from build123d import *

# Parameters (mm, degrees)
SKETCH1_W                    = 26.140328994
SKETCH1_H                    = 20
BASE_FLANGE1_DEPTH           = 3.175
EDGE_FLANGE1_STRIP_W         = 14.7
EDGE_FLANGE1_STRIP_H         = 3.175
EDGE_FLANGE1_STRIP_CUT_DEPTH = 20
EDGE_FLANGE1_DEPTH           = 20
EDGE_FLANGE2_STRIP_W         = 14.7
EDGE_FLANGE2_STRIP_H         = 3.175
EDGE_FLANGE2_STRIP_CUT_DEPTH = 20
EDGE_FLANGE2_DEPTH           = 20
FILLET1_R                    = 3
SKETCH18_R                   = 2.54
CUT_EXTRUDE2_DEPTH           = 360.816616057
SKETCH19_R                   = 2.54
CUT_EXTRUDE3_DEPTH           = 360.466065193


# Sheet-metal steps are written as plain solids
with BuildPart() as part:
    # Sketch1 → Base-Flange1 (new body)
    with BuildSketch(Plane.XY.offset(-1949.683434301)):
        with Locations((87.899449082, 311.128054742)):
            Rectangle(SKETCH1_W, SKETCH1_H)
    extrude(amount=BASE_FLANGE1_DEPTH)

    # Edge-Flange1 strip (across the edge) → Edge-Flange1 strip cut (cut)
    with BuildSketch(Plane(origin=(100.969613579, 321.128054742, -1949.683434301), x_dir=(-1, 0, 0), z_dir=(0, -1, 0))):
        with Locations((-6.35, -1.5875)):
            Rectangle(EDGE_FLANGE1_STRIP_W, EDGE_FLANGE1_STRIP_H)
    extrude(amount=EDGE_FLANGE1_STRIP_CUT_DEPTH, mode=Mode.SUBTRACT)

    # Edge-Flange1 section (across the edge) → Edge-Flange1 (add)
    with BuildSketch(Plane(origin=(100.969613579, 321.128054742, -1949.683434301), x_dir=(-1, 0, 0), z_dir=(0, -1, 0))):
        with BuildLine():
            Line((-3.175, 1), (-3.175, 34.9454))
            Line((-3.175, 34.9454), (0, 34.9454))
            Line((0, 34.9454), (0, 1))
            ThreePointArc((0, 1), (0.292893219, 0.292893219), (1, 0))
            Line((1, 0), (1, -3.175))
            ThreePointArc((1, -3.175), (-1.952170811, -1.952170811), (-3.175, 1))
        make_face()
    extrude(amount=EDGE_FLANGE1_DEPTH)

    # Edge-Flange2 strip (across the edge) → Edge-Flange2 strip cut (cut)
    with BuildSketch(Plane(origin=(104.144613579, 301.128054742, -1984.628834301), x_dir=(0, 0, 1), z_dir=(0, 1, 0))):
        with Locations((-6.35, -1.5875)):
            Rectangle(EDGE_FLANGE2_STRIP_W, EDGE_FLANGE2_STRIP_H)
    extrude(amount=EDGE_FLANGE2_STRIP_CUT_DEPTH, mode=Mode.SUBTRACT)

    # Edge-Flange2 section (across the edge) → Edge-Flange2 (add)
    with BuildSketch(Plane(origin=(104.144613579, 301.128054742, -1984.628834301), x_dir=(0, 0, 1), z_dir=(0, 1, 0))):
        with BuildLine():
            Line((-3.175, 1), (-3.175, 52.825))
            Line((-3.175, 52.825), (0, 52.825))
            Line((0, 52.825), (0, 1))
            ThreePointArc((0, 1), (0.292893219, 0.292893219), (1, 0))
            Line((1, 0), (1, -3.175))
            ThreePointArc((1, -3.175), (-1.952170811, -1.952170811), (-3.175, 1))
        make_face()
    extrude(amount=EDGE_FLANGE2_DEPTH)

    # Fillet1
    fillet1_edges = [part.edges().sort_by_distance(p)[0] for p in [
        (156.969613579, 301.128054742, -1986.216334301),
        (156.969613579, 321.128054742, -1986.216334301),
        (74.829284585, 301.128054742, -1948.095934301),
        (74.829284585, 321.128054742, -1948.095934301),
    ]]
    fillet(fillet1_edges, radius=FILLET1_R)

    # Sketch18 → Cut-Extrude2 (cut, through all)
    with BuildSketch(Plane.XY.offset(-1946.508434301)):
        with Locations((79.909284585, 311.128054742)):
            Circle(SKETCH18_R)
    extrude(amount=-CUT_EXTRUDE2_DEPTH, mode=Mode.SUBTRACT)

    # Sketch19 → Cut-Extrude3 (cut, through all)
    with BuildSketch(Plane.XY.offset(-1984.628834301)):
        with Locations((151.889613579, 311.128054742)):
            Circle(SKETCH19_R)
    extrude(amount=-CUT_EXTRUDE3_DEPTH, mode=Mode.SUBTRACT)


solid = part.part
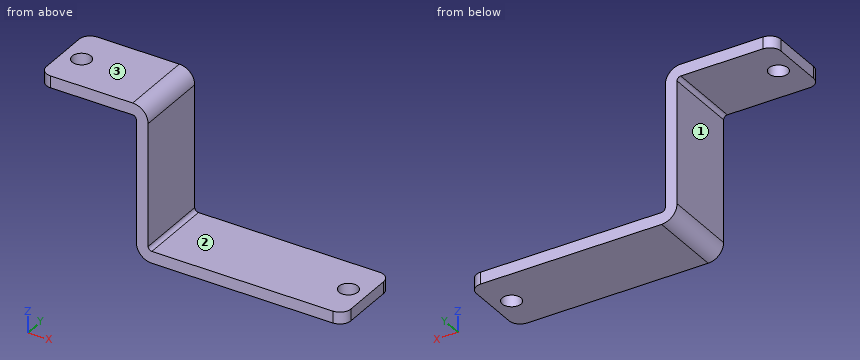
Part model, mm, in its own coordinate system. Face numbers are marked on the shaded views. A direction names the side the tool comes from. Coordinates: 2 decimals unless noted, no trailing zeros. Order: outer loops, then holes, each group sorted by start corner. A loop starts at its lowest first (then second) coordinate and runs counter-clockwise, first axis right, second up.
(1) Slice it at D-D, the plane x = 94. Write the cut outline in (y, z).
Check sheet entries:
outline: (301.13, -1949.68) - (321.13, -1949.68) - (321.13, -1946.51) - (301.13, -1946.51) - close
(2) Pin check, flat tips, straight feed: pin 1 Ø6 at (x, y) = (142.5, 314.5) entering from +Z; pin 2 Ø12 at (y, z) = (315, -1969.5) entering from +X; pin 3 Ø6 at (x, y) = (84, 307.5) entering from -Z. Stop position of each tip, or through.
Check sheet entries:
pin 1: stops at z = -1984.63
pin 2: stops at x = 104.14
pin 3: stops at z = -1949.68
(3) Slice it at B-B, the plane y = 314.5. Write the cut outline in (x, z) (3 decimals).
Check sheet entries:
outline: (74.829, -1949.683) - (99.97, -1949.683) arc R1 cw to (100.97, -1950.683) - (100.97, -1983.629) arc R4.175 ccw to (105.145, -1987.804) - (156.97, -1987.804) - (156.97, -1984.629) - (105.145, -1984.629) arc R1 cw to (104.145, -1983.629) - (104.145, -1950.683) arc R4.175 ccw to (99.97, -1946.508) - (74.829, -1946.508) - close
(4) Tool access for the marked faces 1, 2 and 3: list every direction of +Z, -Z, +X, -X, +Y, -Y with a clear straight run to the whole face (end or side of a thin tool).
Check sheet entries:
face 1: -Z, -X, +Y, -Y
face 2: +Z, +X, +Y, -Y
face 3: +Z, +X, -X, +Y, -Y
(5) Probe L1, parallel to Z at x = 125.5, y = 313.25; L2, parallel to X at y = 313.5, z = -1955.5; L3, parallel to Z at x = 89, y = 311.75. List the from-to ranges inside material, lowest first.
Check sheet entries:
L1: z = -1987.8 to -1984.63
L2: x = 100.97 to 104.14
L3: z = -1949.68 to -1946.51
(6) Slice it at A-A, the plane x = 81. Write the cut outline in (y, z).
Check sheet entries:
outline: (301.13, -1949.68) - (308.83, -1949.68) - (308.83, -1946.51) - (301.13, -1946.51) - close; (313.42, -1949.68) - (321.13, -1949.68) - (321.13, -1946.51) - (313.42, -1946.51) - close
(7) Slice it at C-C, the plane z = -1966. Write the cut outline in (x, y), and give its area (3 significant figures).
Check sheet entries:
outline: (100.97, 301.13) - (104.14, 301.13) - (104.14, 321.13) - (100.97, 321.13) - close
area: 63.5 mm2
